Here's how the part is built. I have some questions about the finished solid (model axes, mm). A direction names the side the tool comes from. Give positions to 0.01 mm unless a question says otherwise; leave off trailing zeros. Use one line per item in the form item = value. Start each with the question number.
from build123d import *

# Parameters (mm, degrees)
BOSS_EXTRUDE1_DEPTH     = 18
SKETCH3_W               = 33
SKETCH3_H               = 10
CUT_EXTRUDE1_DEPTH      = 143.562267098
CUT_EXTRUDE2_DEPTH      = 143.562267098
CUT_EXTRUDE3_DEPTH      = 143.562267098
CUT_EXTRUDE4_DEPTH      = 143.562267098
BOSS_EXTRUDE2_DEPTH     = 18
BOSS_EXTRUDE3_DEPTH     = 18
LPATTERN1_COUNT         = 30
LPATTERN1_PITCH         = 3
CUT_EXTRUDE5_DEPTH      = 146.668613805
CUT_EXTRUDE6_DEPTH      = 146.668613805
CUT_EXTRUDE7_DEPTH      = 146.668613805
CUT_EXTRUDE8_DEPTH      = 146.668613805
FILLET1_R               = 5
F_6_0_MM_DOWEL_HOLES1_D = 6.2


with BuildPart() as part:
    # Sketch2 → Boss-Extrude1 (new body)
    with BuildSketch(Plane.XY):
        with BuildLine():
            Line((-20, 0), (20, 0))
            Line((20, 0), (20, 140))
            ThreePointArc((20, 140), (-9.083269132, 116.055512755), (-20, 80))
            Line((-20, 80), (-20, 0))
        make_face()
    extrude(amount=BOSS_EXTRUDE1_DEPTH)

    # Sketch3 → Cut-Extrude1 (cut, through all)
    with BuildSketch(Plane.XY.offset(18)):
        with Locations((0.5, 28)):
            Rectangle(SKETCH3_W, SKETCH3_H)
    extrude(amount=-CUT_EXTRUDE1_DEPTH, mode=Mode.SUBTRACT)

    # Sketch4 → Cut-Extrude2 (cut, through all)
    with BuildSketch(Plane.XY.offset(18)):
        Polygon((-16, 36), (17, 36), (17, 46), (-16, 51.818790363), align=None)
    extrude(amount=-CUT_EXTRUDE2_DEPTH, mode=Mode.SUBTRACT)

    # Sketch5 → Cut-Extrude3 (cut, through all)
    with BuildSketch(Plane.XY.offset(18)):
        Polygon((-16, 54.865070199), (17, 49.046279836), (17, 59.046279836), (-16, 71.057297566), align=None)
    extrude(amount=-CUT_EXTRUDE3_DEPTH, mode=Mode.SUBTRACT)

    # Sketch6 → Cut-Extrude4 (cut, through all)
    with BuildSketch(Plane.XY.offset(18)):
        with BuildLine():
            Line((-16, 74.249830884), (17, 62.238813153))
            Line((17, 62.238813153), (17, 72.238813153))
            Line((17, 72.238813153), (-15.046889298, 90.741093316))
            ThreePointArc((-15.046889298, 90.741093316), (-15.761255119, 85.391648765), (-16, 80))
            Line((-16, 80), (-16, 74.249830884))
        make_face()
    extrude(amount=-CUT_EXTRUDE4_DEPTH, mode=Mode.SUBTRACT)

    # Sketch13 → Boss-Extrude2 (add)
    with BuildSketch(Plane.XY.offset(18)):
        with BuildLine():
            Line((27.463865989, 141.919276749), (27.463865989, 139.919276749))
            ThreePointArc((27.463865989, 139.919276749), (21.883638711, 121.290161062), (20, 101.934676234))
            Line((20, 101.934676234), (20, 140))
            ThreePointArc((20, 140), (23.663152719, 141.227117654), (27.463865989, 141.919276749))
        make_face()
    extrude(amount=-BOSS_EXTRUDE2_DEPTH)

    # Sketch15 → Boss-Extrude3 (add)
    with BuildSketch(Plane.XY.offset(18)):
        Polygon((20, 101.934676234), (22.598076211, 100.434676234), (20, 98.934676234), align=None)
    boss_extrude3 = extrude(amount=-BOSS_EXTRUDE3_DEPTH)

    # LPattern1: Boss-Extrude3 ×30
    with Locations(*[(0, -i * LPATTERN1_PITCH, 0) for i in range(1, LPATTERN1_COUNT)]):
        add(boss_extrude3)

    # Sketch17 → Cut-Extrude5 (cut, through all)
    with BuildSketch(Plane.XY.offset(18)):
        with BuildLine():
            Line((-14.409820926, 93.837383335), (17, 75.702914768))
            Line((17, 75.702914768), (17, 85.702914768))
            Line((17, 85.702914768), (-9.308172311, 107.778092451))
            ThreePointArc((-9.308172311, 107.778092451), (-12.284651864, 100.963507838), (-14.409820926, 93.837383335))
        make_face()
    extrude(amount=-CUT_EXTRUDE5_DEPTH, mode=Mode.SUBTRACT)

    # Sketch18 → Cut-Extrude6 (cut, through all)
    with BuildSketch(Plane.XY.offset(18)):
        with BuildLine():
            Line((-7.846238812, 110.46760646), (17, 89.619136636))
            Line((17, 89.619136636), (17, 99.619136636))
            Line((17, 99.619136636), (-0.566824758, 120.554463152))
            ThreePointArc((-0.566824758, 120.554463152), (-4.464319866, 115.697073553), (-7.846238812, 110.46760646))
        make_face()
    extrude(amount=-CUT_EXTRUDE6_DEPTH, mode=Mode.SUBTRACT)

    # Sketch19 → Cut-Extrude7 (cut, through all)
    with BuildSketch(Plane.XY.offset(18)):
        with BuildLine():
            Line((1.497556464, 122.761400894), (17, 104.286308117))
            Line((17, 104.286308117), (17, 114.286308117))
            Line((17, 114.286308117), (8.554035532, 128.915147695))
            ThreePointArc((8.554035532, 128.915147695), (4.907555132, 125.973860666), (1.497556464, 122.761400894))
        make_face()
    extrude(amount=-CUT_EXTRUDE7_DEPTH, mode=Mode.SUBTRACT)

    # Sketch21 → Cut-Extrude8 (cut, through all)
    with BuildSketch(Plane.XY.offset(18)):
        with BuildLine():
            Line((11.013641865, 130.654984559), (17, 120.286308117))
            Line((17, 120.286308117), (17, 134.194095619))
            ThreePointArc((17, 134.194095619), (13.956345649, 132.509918344), (11.013641865, 130.654984559))
        make_face()
    extrude(amount=-CUT_EXTRUDE8_DEPTH, mode=Mode.SUBTRACT)

    # Fillet1
    fillet1_edges = [part.edges().sort_by_distance(p)[0] for p in [
        (20, 0, 9),
        (-20, 0, 9),
    ]]
    fillet(fillet1_edges, radius=FILLET1_R)

    # Ø6.0 mm Dowel Holes1 (through all)
    with Locations(Plane.XY.offset(18)):
        with Locations((-15, 5)):
            f_6_0_mm_dowel_holes1 = Hole(F_6_0_MM_DOWEL_HOLES1_D / 2)

    # Mirror1: Ø6.0 mm Dowel Holes1 across plane
    add(f_6_0_mm_dowel_holes1.mirror(Plane(origin=(0, 0, 0), x_dir=(0, 0, 1), z_dir=(1, 0, 0))), mode=Mode.SUBTRACT)


solid = part.part
1) Thinking about a two-plate mould opening in Y: for faces 3 (the face through (-19, 2, 9)), 4 (the face through (21.281, 38.195, 9.126)), 5 (the face through (-20, 43, 9)), which applies, released by +Y, released by -Y, zero draft, split by the parting line, or undercut?
2) On a 3-axis mill with a long thin cutter (end or side, diameter ignored), from which of +Z, -Z, +X, -X, +Y, -Y can I reach the whole of each face in a straight line? I mean faces 1 (the face through (21.281, 101.195, 9.126)), 2 (the face through (8.34, 109.94, 9.13)). Say none if no direction works.
3) Suppose I cut it at A-A, the plane x = 3.5. State how many separate pieces and enclosed holes the cut face has, and give its area (3 significant figures).
4) Please list where these lines run through material, in increasing order: line 1 (Y direction, x = -15, z = 6.5); line 2 (Y direction, x = -8, z = 2.25); line 3 (X direction, y = 79.5, z = 4).
5) Will these pins go through, and if not, where does the flat tip stop? P1, Ø6, axis at y = 37.5, z = 10.5, coming from the +X side; P2, Ø7.5, axis at y = 8, z = 5.5, coming from the +X side; P3, Ø4, axis at x = 19, z = 2, coming from the +Y side.
Checks:
q1.face_3 = released by -Y
q1.face_4 = undercut
q1.face_5 = zero draft
q2.face_1 = +Z, -Z, +X
q2.face_2 = +Z, -Z
q3.separate_pieces = 8
q3.enclosed_holes = 0
q3.area = 893 mm^2
q4.line_1 = 0 to 1.9, 8.1 to 23, 33 to 36, 51.64 to 54.69, 70.69 to 73.89, 90.71 to 105
q4.line_2 = 0 to 23, 33 to 36, 50.41 to 53.45, 68.15 to 71.34, 86.67 to 90.14, 106.68 to 117.63
q4.line_3 = -20 to -16, 4.42 to 10.42, 17 to 22.48
q5.P1 = 22.6
q5.P2 = 20
q5.P3 = 140.39
